Source: CAD feature listing. Evaluate the final solid. Frame: model axes, mm. Face numbers are marked on the shaded views. A direction names the side the tool comes from. Give positions to 0.01 mm unless a question says otherwise; leave off trailing zeros. Order: outer loops, then holes, each group sorted by start corner. A loop starts at its lowest first (then second) coordinate and runs counter-clockwise, first axis right, second up. Notation, with made-up numbers: M 40.5,71 L 93.5,71 A16 ccw 93.5,96 Z; hole C 55,62.25 d1. An arc over 180 degrees is marked long. Use CSV: the item, a comma, the result in double quotes. Start each with the question number.
1. Reachability of the marked faces 1, 2 and 3 from +Z, -Z, +X, -X, +Y, -Y: full face, straight path, thin tool, end or side. Return the list, or none.
2. Line query: line 1 along Z through (x, y) = (29, -3.75); line 2 along X through (y, z) = (8.25, -2.5); line 3 along X through (y, z) = (-3, -4.5). Output: solid intervals per line, ascending. Write a range as [from, to].
3. Section query B-B, the plane y = -1.5. Return the cut outline in (x, z), plus the area to 3 significant figures.
4. Section query D-D, the plane x = 23. Return the cut outline in (y, z), plus the area to 3 significant figures.
5. Section query A-A, the plane z = -6.5. Return the cut outline in (x, y).
6. Pin query (flat end, axial travel): P1, Ø2, axis at y = 6, z = -25.5, coming from the +X side; P2, Ø1, axis at x = 0, y = 3.5, coming from the +Z side; P3, Ø1.5, axis at x = 44.5, z = -2, coming from the +Y side. Return the tip coordinate at first contact, or that it passes through.
7. Section query C-C, the plane y = 8.5. Return the cut outline in (x, z), plus the area to 3 significant figures.
from build123d import *

# Parameters (mm, degrees)
BOSS_EXTRUDE1_DEPTH      = 10
BOSS_EXTRUDE1_DEPTH_BACK = 10
SKETCH2_R                = 2.5
CUT_EXTRUDE1_DEPTH       = 4
SPLIT2_SURFACE_1_BACK    = 108.282
SPLIT2_SURFACE_1_DEPTH   = 216.564


with BuildPart() as part:
    # Sketch1 → Boss-Extrude1 (new, two sides)
    with BuildSketch(Plane(origin=(0, 0, 0), x_dir=(1, 0, 0), z_dir=(0, 1, 0))) as boss_extrude1_sk:
        Polygon((-51.374196063, 7.601926758), (-51.374196063, -2.398073242), (-41.374196063, -2.398073242), (-41.374196063, 3.123704189), (-21.449234595, 20.908790051), (4.969602102, 20.908790051), (23.858490991, -2.398073242), (48.625803937, -2.398073242), (48.625803937, 7.601926758), (28.625803937, 7.601926758), (9.736915048, 30.908790051), (-25.263084952, 30.908790051), align=None)
    extrude(amount=BOSS_EXTRUDE1_DEPTH)
    extrude(boss_extrude1_sk.sketch, amount=-BOSS_EXTRUDE1_DEPTH_BACK)

    # Sketch2 → Cut-Extrude1 (cut)
    with BuildSketch(Plane(origin=(0, 10, 0), x_dir=(1, 0, 0), z_dir=(0, 1, 0))):
        with Locations(Location((45.625803937, 2.601926758, 0), (0, 0, 270))):
            Circle(SKETCH2_R)
    extrude(amount=-CUT_EXTRUDE1_DEPTH, mode=Mode.SUBTRACT)

    # Split2: cut with a surface, the side behind it stays
    # Split2 surface: a surface, the sketch's curves swept straight by 216.564 mm
    with BuildLine(Plane(origin=(0, -10, 0), x_dir=(-1, 0, 0), z_dir=(0, -1, 0)).offset(-SPLIT2_SURFACE_1_BACK), mode=Mode.PRIVATE) as split2_surface_1_path:
        Line((51.374196063, 7.601926758), (41.374196063, 3.123704189))
    split2_surface_1 = Shell.extrude(split2_surface_1_path.wire(), (0 * SPLIT2_SURFACE_1_DEPTH, -1 * SPLIT2_SURFACE_1_DEPTH, 0 * SPLIT2_SURFACE_1_DEPTH))
    split(bisect_by=split2_surface_1, keep=Keep.BOTTOM)


solid = part.part
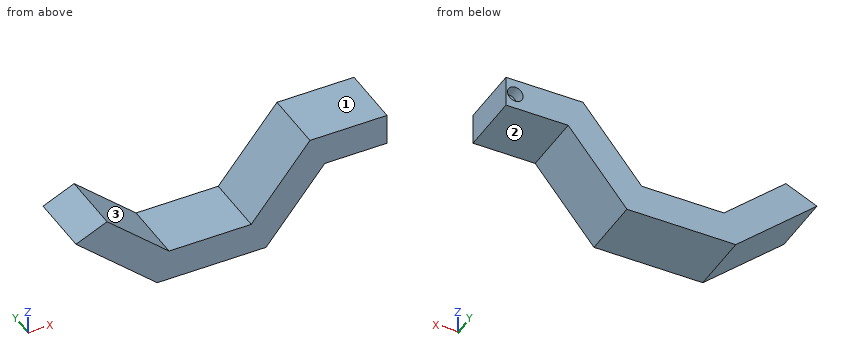
Result set:
1,face 1,"+Z, +X, -X, +Y, -Y"
1,face 2,"-Z, +X, +Y, -Y"
1,face 3,"+Z, +Y, -Y"
2,line 1,"[-7.6, 2.4]"
2,line 2,"[19.89, 43.13], [48.12, 48.63]"
2,line 3,"[-44.45, -39.83], [18.27, 48.63]"
3,outline,"M -51.37,-7.6 L -25.26,-30.91 L 9.74,-30.91 L 28.63,-7.6 L 48.63,-7.6 L 48.63,2.4 L 23.86,2.4 L 4.97,-20.91 L -21.45,-20.91 L -41.37,-3.12 Z"
3,area,"1,140 mm2"
4,outline,"M -10,-14.54 L 10,-14.54 L 10,1.34 L -10,1.34 Z"
4,area,"318 mm2"
5,outline,"M -48.91,-10 L -37.59,-10 L -37.59,10 L -48.91,10 Z; M 16.65,-10 L 48.63,-10 L 48.63,10 L 16.65,10 Z"
6,P1,"x = 14.93"
6,P2,"z = -20.91"
6,P3,"y = 6"
7,outline,"M -51.37,-7.6 L -25.26,-30.91 L 9.74,-30.91 L 28.63,-7.6 L 48.63,-7.6 L 48.63,2.4 L 23.86,2.4 L 4.97,-20.91 L -21.45,-20.91 L -41.37,-3.12 Z; hole C 45.63,-2.6 d5"
7,area,"1,120 mm2"
